from build123d import *

# Parameters (mm, degrees)
CROQUIS1_W              = 19.8
CROQUIS1_H              = 11.5
SALIENTE_EXTRUIR1_DEPTH = 70.5
VACIADO1_T              = -2
CROQUIS4_W              = 15.8
CROQUIS4_H              = 28
CORTAR_EXTRUIR1_DEPTH   = 2
REDONDEO1_R             = 8
CROQUIS5_W              = 15.8
CROQUIS5_H              = 2
SALIENTE_EXTRUIR2_DEPTH = 2
CROQUIS6_W              = 19.8
CROQUIS6_H              = 8
SALIENTE_EXTRUIR4_DEPTH = 16
CROQUIS8_R              = 1
CORTAR_EXTRUIR3_DEPTH   = 10
SALIENTE_EXTRUIR5_DEPTH = 19.8
CROQUIS10_R             = 3.1
CORTAR_EXTRUIR4_DEPTH   = 19.8


with BuildPart() as part:
    # Croquis1 → Saliente-Extruir1 (new body)
    with BuildSketch(Plane(origin=(0, 0, 0), x_dir=(0, 1, 0), z_dir=(0, 0, 1))):
        Rectangle(CROQUIS1_W, CROQUIS1_H)
    extrude(amount=SALIENTE_EXTRUIR1_DEPTH)

    # Vaciado1
    vaciado1_openings = [part.faces().sort_by_distance(p)[0] for p in [
        (0, 0, 70.5),
    ]]
    offset(amount=VACIADO1_T, openings=vaciado1_openings, kind=Kind.INTERSECTION)

    # Croquis4 → Cortar-Extruir1 (cut)
    with BuildSketch(Plane.YZ.offset(5.75)):
        with Locations((0, 56.5)):
            Rectangle(CROQUIS4_W, CROQUIS4_H)
    extrude(amount=-CORTAR_EXTRUIR1_DEPTH, mode=Mode.SUBTRACT)

    # Redondeo1
    # the kernel refuses this fillet: 8 mm, written as the material it adds along each edge
    with BuildSketch(Plane(origin=(5.75, 7.9, 42.5), x_dir=(0, -1, 0), z_dir=(-1, 0, 0)), Plane(origin=(5.75, -7.9, 42.5), x_dir=(0, 0, 1), z_dir=(-1, 0, 0))) as redondeo1_piece_1:
        with BuildLine():
            CenterArc((REDONDEO1_R, REDONDEO1_R), REDONDEO1_R, 180, 90)
            Line((0, REDONDEO1_R), (0, 0))
            Line((0, 0), (REDONDEO1_R, 0))
        make_face()
    extrude(amount=2)

    # Croquis5 → Saliente-Extruir2 (add)
    with BuildSketch(Plane.YZ.offset(5.75)):
        with Locations((0, 69.5)):
            Rectangle(CROQUIS5_W, CROQUIS5_H)
    extrude(amount=-SALIENTE_EXTRUIR2_DEPTH)

    # Croquis6 → Saliente-Extruir4 (add)
    with BuildSketch(Plane(origin=(-5.75, 0, 0), x_dir=(0, -1, 0), z_dir=(-1, 0, 0))):
        with Locations((0, 24)):
            Rectangle(CROQUIS6_W, CROQUIS6_H)
    extrude(amount=SALIENTE_EXTRUIR4_DEPTH)

    # Croquis8 → Cortar-Extruir3 (cut)
    with BuildSketch(Plane.XY.offset(28)):
        with Locations((-16.75, 4.9)):
            Circle(CROQUIS8_R)
        with Locations((-16.75, -4.9)):
            Circle(CROQUIS8_R)
    extrude(amount=-CORTAR_EXTRUIR3_DEPTH, mode=Mode.SUBTRACT)

    # Croquis9 → Saliente-Extruir5 (add)
    with BuildSketch(Plane.XZ.offset(9.9)):
        Polygon((-5.75, 70.5), (-13.75, 28), (-5.75, 28), align=None)
        Polygon((-5.75, 0), (-13.75, 20), (-5.75, 20), align=None)
    extrude(amount=-SALIENTE_EXTRUIR5_DEPTH)

    # Croquis10 → Cortar-Extruir4 (cut)
    with BuildSketch(Plane.XZ.offset(9.9)):
        with Locations(Location((-16.745253682, 24, 0), (0, 0, 270))):
            Circle(CROQUIS10_R)
    extrude(amount=-CORTAR_EXTRUIR4_DEPTH, mode=Mode.SUBTRACT)


solid = part.part
Geometry: final body of the model. Coordinates: model frame, mm. A direction names the side the tool comes from. Round coordinates to 2 decimals unless told otherwise and drop trailing zeros. Order: outer loops, then holes, each group sorted by start corner. A loop starts at its lowest first (then second) coordinate and runs counter-clockwise, first axis right, second up.
Q1. Material intervals for probe 1 along X at (y, z) = (-4.9, 27.75); probe 2 along Y at (x, z) = (-16.75, 27.5); probe 3 along Y at (x, z) = (-0.25, 56.5), sorted ascending.
Result sheet:
probe 1: x = -21.75 to -17.75, -15.75 to -3.75, 3.75 to 5.75
probe 2: y = -9.9 to -5.9, -3.9 to 3.9, 5.9 to 9.9
probe 3: y = -9.9 to -7.9, 7.9 to 9.9
Q2. Section B-B, the plane y = 2.75. Output: boundary loops of the cut face in (x, z).
Result sheet:
outline: (-21.75, 20) - (-13.75, 20) - (-5.75, 0) - (5.75, 0) - (5.75, 43.02) - (3.75, 43.02) - (3.75, 2) - (-3.75, 2) - (-3.75, 70.5) - (-5.75, 70.5) - (-13.75, 28) - (-21.75, 28) - close; (3.75, 68.5) - (5.75, 68.5) - (5.75, 70.5) - (3.75, 70.5) - close; hole circle Ø6.2 at (-16.75, 24)
Q3. Access query for faces 4 (the face through (4.76, 5.65, 44.94)), 5 (the face through (5.75, 0, 28)), 6 (the face through (-18, 0, 28)), 7 (the face through (-15.796, -4.6, 20.541)), 8 (the face through (3.75, 0, 70)). Directions: +Z, -Z, +X, -X, +Y, -Y. A direction counts if a zero-diameter tool reaches every point of the face in a straight line with its end or side. Return the directions, or none.
Result sheet:
face 4: +X
face 5: +Z, -Z, +X, +Y, -Y
face 6: +Z, -X, +Y, -Y
face 7: +Z, -Z
face 8: +Z
Q4. Pin query (flat end, axial travel): pin 1 (2 mm diameter, centred on x = -2, y = -0.5, fed in from +Z); pin 2 (12 mm diameter, centred on x = -10, z = 52.5, fed in from -Y); pin 3 (2.5 mm diameter, centred on x = -16.75, y = -4.9, fed in from +Z); pin 4 (1.8 mm diameter, centred on x = -16.75, y = 4.9, fed in from -Z). Return the tip coordinate at first contact, or that it passes through.
Result sheet:
pin 1: stops at z = 2
pin 2: stops at y = -9.9
pin 3: stops at z = 28
pin 4: passes through
Q5. Section A-A, the plane z = 24. Output: boundary loops of the cut face in (x, y), and give its area (3 significant figures).
Result sheet:
outline: (-21.75, -9.9) - (-19.85, -9.9) - (-19.85, 9.9) - (-21.75, 9.9) - close; (-13.65, -9.9) - (5.75, -9.9) - (5.75, 9.9) - (-13.65, 9.9) - close; hole (-3.75, -7.9) - (3.75, -7.9) - (3.75, 7.9) - (-3.75, 7.9) - close
area: 303 mm2
Q6. Section D-D, the plane x = 2. Output: boundary loops of the cut face in (y, z).
Result sheet:
outline: (-9.9, 0) - (9.9, 0) - (9.9, 70.5) - (7.9, 70.5) - (7.9, 2) - (-7.9, 2) - (-7.9, 70.5) - (-9.9, 70.5) - close
Q7. Section C-C, the plane z = 16. Output: boundary loops of the cut face in (x, y).
Result sheet:
outline: (-12.15, -9.9) - (5.75, -9.9) - (5.75, 9.9) - (-12.15, 9.9) - close; hole (-3.75, -7.9) - (3.75, -7.9) - (3.75, 7.9) - (-3.75, 7.9) - close
Q8. Mould query, pull axis Z, two halves, no side actions, for faces 1 (the face through (3.75, 0, 21)), 2 (the face through (5, 0, 68.5)), 3 (the face through (-9.694, -0.139, 49.548)). Classes: released by +Z, released by -Z, zero draft, split by the parting line, or undercut.
Result sheet:
face 1: zero draft
face 2: undercut
face 3: released by +Z
